```python
from build123d import *

# Parameters (mm, degrees)
EXTRUDE_1_DEPTH     = 25
SKETCH_2_R          = 3.2
CUT_EXTRUDE_1_DEPTH = 35
SKETCH_3_R          = 3.2
CUT_EXTRUDE_2_DEPTH = 35


with BuildPart() as part:
    # 스케치1 → 보스-돌출1 (new body)
    with BuildSketch(Plane(origin=(0, 0, 0), x_dir=(1, 0, 0), z_dir=(0, 1, 0))):
        Polygon((-17.5, 79.05), (-11.25, 79.05), (-11.25, 49.05), (11.25, 49.05), (11.25, 79.05), (17.5, 79.05), (17.5, -17.5), (-79.05, -17.5), (-79.05, -11.25), (-49.05, -11.25), (-49.05, 11.25), (-79.05, 11.25), (-79.05, 17.5), (-17.5, 17.5), align=None)
    extrude(amount=EXTRUDE_1_DEPTH)

    # 스케치2 → 컷-돌출1 (cut)
    with BuildSketch(Plane(origin=(17.5, 0, 0), x_dir=(0, 0, -1), z_dir=(1, 0, 0))):
        with Locations((71.55, 12.5)):
            Circle(SKETCH_2_R)
        with Locations((56.55, 12.5)):
            Circle(SKETCH_2_R)
    extrude(amount=-CUT_EXTRUDE_1_DEPTH, mode=Mode.SUBTRACT)

    # 스케치3 → 컷-돌출2 (cut)
    with BuildSketch(Plane.XY.offset(17.5)):
        with Locations((-71.55, 12.5)):
            Circle(SKETCH_3_R)
        with Locations((-56.55, 12.5)):
            Circle(SKETCH_3_R)
    extrude(amount=-CUT_EXTRUDE_2_DEPTH, mode=Mode.SUBTRACT)


solid = part.part
```
Part model, mm, in its own coordinate system. A direction names the side the tool comes from. Give positions to 0.01 mm unless a question says otherwise; leave off trailing zeros. Order: outer loops, then holes, each group sorted by start corner. A loop starts at its lowest first (then second) coordinate and runs counter-clockwise, first axis right, second up. Notation, with made-up numbers: M 70,-29.5 L 125,-29.5 A31 ccw 125,3.5 Z; hole C -17,75 d11. An arc over 180 degrees is marked long. Use a Markdown table: item, result. Add a question column.
(1) Saw through at C-C, the plane x = -51. Give the cut face in (y, z).
(2) Saw through at D-D, the plane y = 19.25. Give the cut face in (x, z).
(3) Mould opens along Z. For faces 4 (the face through (-30, 12, 17.5)), 5 (the face through (17.5, 12, -31)), 6 (the face through (-14.331, 9.376, -70.856)) say: +Z half, -Z half, draft (parallel to the pull), parting line (faces both ways), or undercut.
(4) Probe line 1 along Z through (x, y) = (-51, 18); line 2 along Y through (x, z) = (-13.75, -56.55); line 3 along Z through (x, y) = (-14, 14.25). List the from-to ranges inside material, lowest first. Write a range as [from, to].
(5) Saw through at B-B, the plane z = -67. Give the cut face in (x, y).
(6) Drop flat-ended pins along their axis: P1, Ø5, axis at y = 12.5, z = -71.55, coming from the -X side; P2, Ø7.5, axis at y = 10.5, z = -64.5, coming from the -X side; P3, Ø11, axis at x = -3.5, y = 7, coming from the -Z side; P4, Ø7.5, axis at x = -56.55, y = 12.5, coming from the -Z side. Give the stop position or say it passes through.
(7) 3-axis set-ups, long thin cutter, end or side, ignore diameter. For faces 1 (the face through (0, 12, -49.05)), 2 (the face through (-49, 12, -17.5)), 3 (the face through (-64, 12, 11.25)): which of +Z, -Z, +X, -X, +Y, -Y reach the whole face in a straight line?
(8) Saw through at A-A, the plane x = -71.55. Give the cut face in (y, z), and give its area (4 significant figures).
Answer key:
| question | item | result |
|---|---|---|
| 1 | outline | M 0,-17.5 L 25,-17.5 L 25,-11.25 L 0,-11.25 Z; M 0,11.25 L 25,11.25 L 25,17.5 L 0,17.5 Z |
| 2 | outline | M -79.05,-17.5 L -17.5,-17.5 L -17.5,-79.05 L -11.25,-79.05 L -11.25,-49.05 L 11.25,-49.05 L 11.25,-79.05 L 17.5,-79.05 L 17.5,17.5 L -79.05,17.5 L -79.05,11.25 L -49.05,11.25 L -49.05,-11.25 L -79.05,-11.25 Z |
| 3 | face 4 | +Z half |
| 3 | face 5 | draft |
| 3 | face 6 | undercut |
| 4 | line 1 | [-17.5, -11.25], [11.25, 17.5] |
| 4 | line 2 | [0, 9.3], [15.7, 25] |
| 4 | line 3 | [-79.05, -74.23], [-68.87, -59.23], [-53.87, 17.5] |
| 5 | outline | M -17.5,0 L -11.25,0 L -11.25,25 L -17.5,25 Z; M 11.25,0 L 17.5,0 L 17.5,25 L 11.25,25 Z |
| 6 | P1 | through |
| 6 | P2 | x = -17.5 |
| 6 | P3 | z = -49.05 |
| 6 | P4 | z = -17.5 |
| 7 | face 1 | -Z, +Y, -Y |
| 7 | face 2 | -Z, -X, +Y, -Y |
| 7 | face 3 | -X, +Y, -Y |
| 8 | outline | M 0,-17.5 L 9.3,-17.5 L 9.3,-11.25 L 0,-11.25 Z; M 0,11.25 L 9.3,11.25 L 9.3,17.5 L 0,17.5 Z; M 15.7,-17.5 L 25,-17.5 L 25,-11.25 L 15.7,-11.25 Z; M 15.7,11.25 L 25,11.25 L 25,17.5 L 15.7,17.5 Z |
| 8 | area | 232.5 mm^2 |
